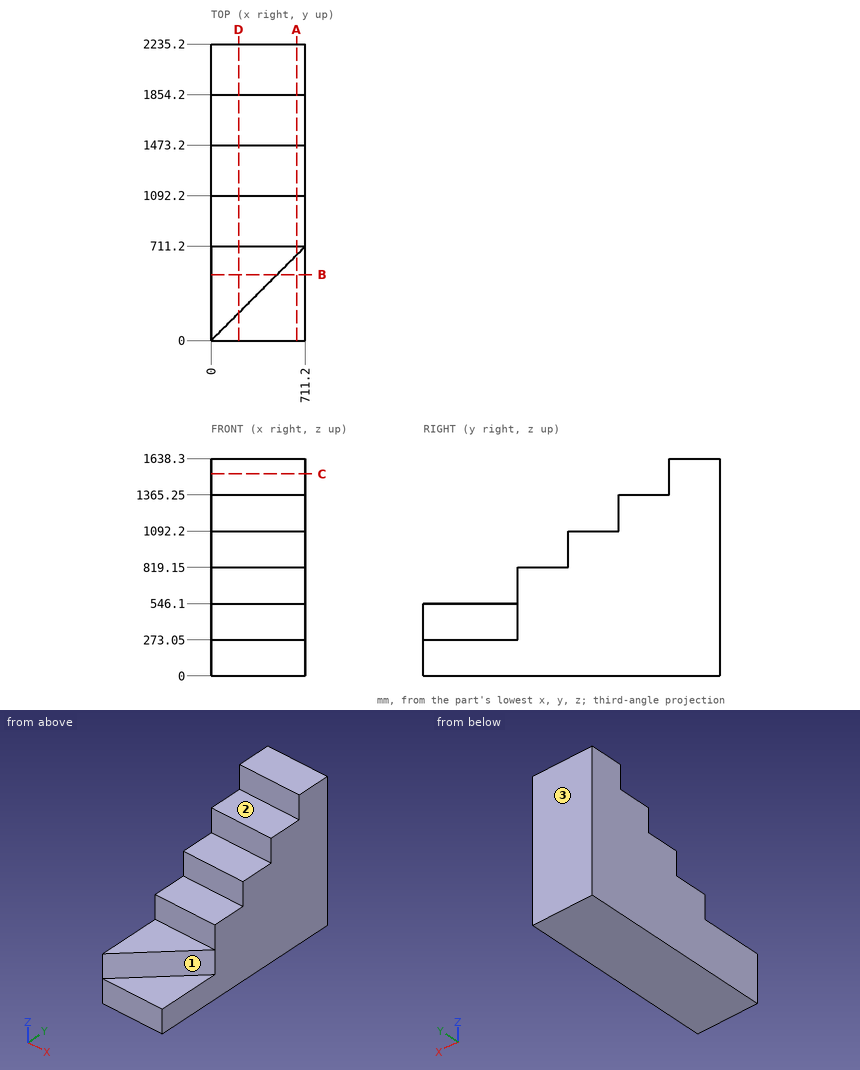
Part print with two shaded views. Sizes in mm from the minimum x, y, z corner. A direction names the side the tool comes from. Coordinates: 2 decimals unless noted, no trailing zeros. Order: outer loops, then holes, each group sorted by start corner. A loop starts at its lowest first (then second) coordinate and runs counter-clockwise, first axis right, second up. Notation, with made-up numbers: M 65,65 L 109,65 A5 ccw 109,74 Z; hole C 69.5,41.5 d11. An arc over 180 degrees is marked long. One line per question, with ' | ' between items. Start each with the question number.
1. Cut at A-A (x = 646). Write the cut outline in (y, z).
2. Flat gauge pins, fed straight in: P1, Ø12, axis at y = 649, z = 436, coming from the +X side; P2, Ø10, axis at x = 137.5, z = 1175, coming from the -Y side. Where does each tip first touch, or does it go through?
3. Wall check: line 1 along Z through (x, y) = (163.5, 104); line 2 along Z through (x, y) = (208, 587.5); line 3 along Y through (x, z) = (407, 1127.5). Give the ranges that are in metal, low to high. Write a range as [from, to].
4. Cut at C-C (z = 1523.5). Write the cut outline in (x, y), plus the area to 3 significant figures.
5. Cut at D-D (x = 208). Write the cut outline in (y, z).
6. Tool access for the marked faces 1, 2 and 3: list every direction of +Z, -Z, +X, -X, +Y, -Y with a clear straight run to the whole face (end or side of a thin tool).
7. Cut at B-B (y = 498). Write the cut outline in (x, z).
The answers:
1) outline: M 0,0 L 2235.2,0 L 2235.2,1638.3 L 1854.2,1638.3 L 1854.2,1365.25 L 1473.2,1365.25 L 1473.2,1092.2 L 1092.2,1092.2 L 1092.2,819.15 L 711.2,819.15 L 711.2,546.1 L 646,546.1 L 646,273.05 L 0,273.05 Z
2) P1: stops at x = 655 | P2: stops at y = 1473.2
3) line 1: z = [0, 273.05] | line 2: z = [0, 546.1] | line 3: y = [1473.2, 2235.2]
4) outline: M 0,1854.2 L 711.2,1854.2 L 711.2,2235.2 L 0,2235.2 Z | area: 271,000 mm2
5) outline: M 0,0 L 2235.2,0 L 2235.2,1638.3 L 1854.2,1638.3 L 1854.2,1365.25 L 1473.2,1365.25 L 1473.2,1092.2 L 1092.2,1092.2 L 1092.2,819.15 L 711.2,819.15 L 711.2,546.1 L 208,546.1 L 208,273.05 L 0,273.05 Z
6) face 1: +Z, +X, -Y | face 2: +Z, +X, -X, -Y | face 3: +Z, -Z, +X, -X, +Y
7) outline: M 0,0 L 711.2,0 L 711.2,273.05 L 498,273.05 L 498,546.1 L 0,546.1 Z
